Source: three-view drawing plus pictorial views. Frame: mm from the lowest corner of the part. A direction names the side the tool comes from. Coordinates: 2 decimals unless noted, no trailing zeros. Loops run counter-clockwise (first coordinate to the right, second up) from the corner with the lowest first, then second, coordinate; pieces in that order, holes last. Notation, with made-up numbers: M 43,-21 L 102,-21 A17 cw 102,-15 Z; hole C 7.25,10.5 d7. An arc over 180 degrees is marked long. Use a Markdown table: item, result. Add a question column.
1. Line query: L1, parallel to Y at x = 1.85, z = 1.3; L2, parallel to X at y = 7.5, z = 1.7; L3, parallel to X at y = 8, z = 2.3 (1 decimal). Output: solid intervals per line, ascending. Write a range as [from, to].
2. Pin query (flat end, axial travel): pin 1 (1.5 mm diameter, centred on y = 7, z = 4.5, fed in from +X); pin 2 (2 mm diameter, centred on y = 5.5, z = 1.5, fed in from +X); pin 3 (1.5 mm diameter, centred on x = 3.5, y = 5.5, fed in from -Z). Return the tip coordinate at first contact, or that it passes through.
3. Section B-B on x = 2.75. Output: boundary loops of the cut face in (y, z) (1 decimal).
4. Set-up query: the marked faces 1, 2 and 3. Return all of +Z, -Z, +X, -X, +Y, -Y with unobstructed straight access to the full face (end or side cutting, diameter ignored); none if empty.
5. Draft query along X for the marked faces 4, 5 and 6. Return one class per face: +X half, -X half, draft (parallel to the pull), parting line (faces both ways), or undercut.
6. Section D-D on y = 6.25. Output: boundary loops of the cut face in (x, z).
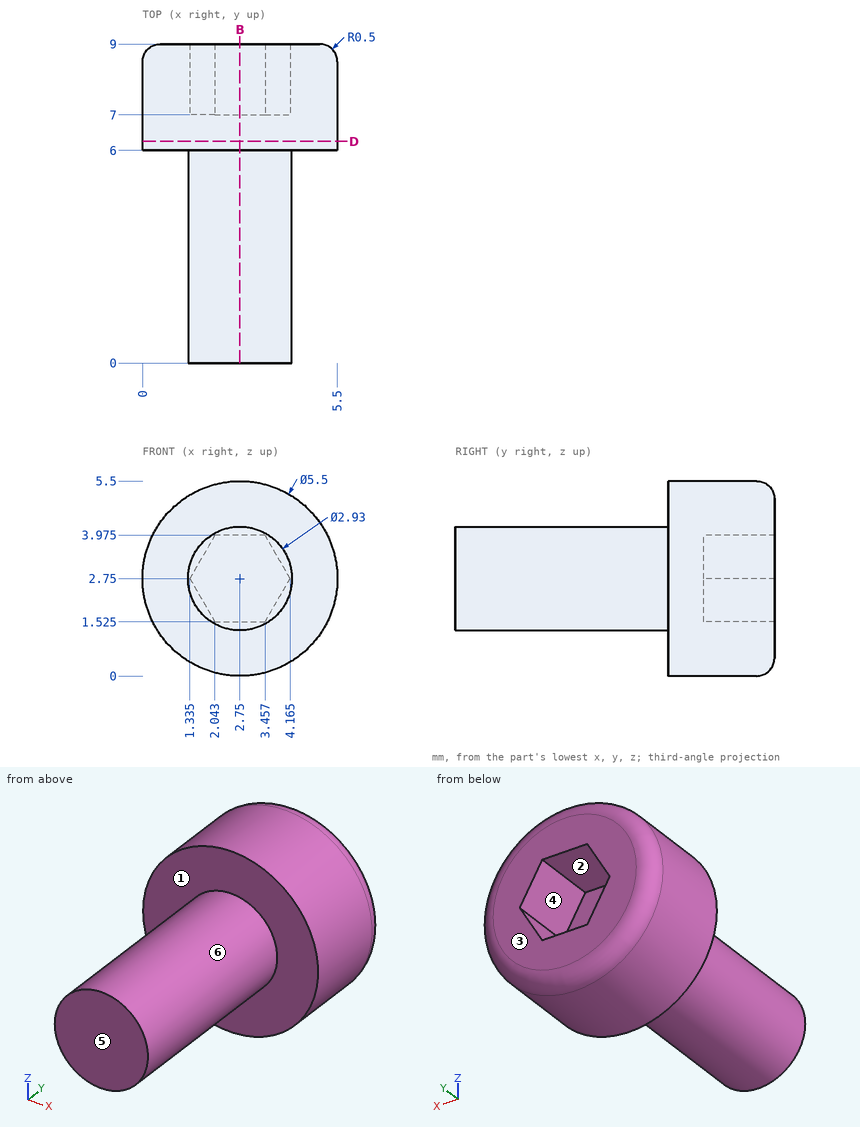
Answers below:
| question | item | result |
|---|---|---|
| 1 | L1 | y = [6, 9] |
| 1 | L2 | x = [0.21, 1.94], [3.56, 5.29] |
| 1 | L3 | x = [0, 1.6], [3.9, 5.5] |
| 2 | pin 1 | stops at x = 5.31 |
| 2 | pin 2 | stops at x = 5.47 |
| 2 | pin 3 | stops at z = 0.01 |
| 3 | outline | M 0,1.3 L 6,1.3 L 6,0 L 8.5,0 A0.5 ccw 9,0.5 L 9,1.5 L 7,1.5 L 7,4 L 9,4 L 9,5 A0.5 ccw 8.5,5.5 L 6,5.5 L 6,4.2 L 0,4.2 Z |
| 4 | face 1 | -Y |
| 4 | face 2 | +Y |
| 4 | face 3 | +Z, -Z, +X, -X, +Y |
| 5 | face 4 | undercut |
| 5 | face 5 | draft |
| 5 | face 6 | parting line |
| 6 | outline | C 2.75,2.75 d5.5 |
